Source: CAD feature listing. Evaluate the final solid. Frame: model axes, mm. A direction names the side the tool comes from. Coordinates: 2 decimals unless noted, no trailing zeros. Order: outer loops, then holes, each group sorted by start corner. A loop starts at its lowest first (then second) coordinate and runs counter-clockwise, first axis right, second up.
Item 1: Ray query, line 1 (Z direction, x = -7.75, y = 0); line 2 (Z direction, x = -7, y = -17); line 3 (Y direction, x = -6.5, z = 27). Return the intervals inside material, ascending.
Item 2: Mould query, pull axis Y, two halves, no side actions, for faces 1 (the flat face through (-5, -1, -18)), 2 (the cylindrical face through (-10.07, 36.4, 0.53)), 3 (the cylindrical face through (-11.796, -17.436, -23.172)), 4 (the cylindrical face through (-3.028, -2.05, -15.616)). Classes: released by +Y, released by -Y, zero draft, split by the parting line, or undercut.
Item 3: Section B-B on z = 0. State how many separate pieces and enclosed holes the cut face has, then the cut area to 3 significant figures.
Item 4: Reachability of faces 5 (the cylindrical face through (-10.06, 40.06, -12.62)), 6 (the cylindrical face through (-11.465, -2.05, 15.616)) from +Z, -Z, +X, -X, +Y, -Y: full face, straight path, thin tool, end or side. Return the list, or none.
Item 5: Section A-A on y = 0. Return the cut outline in (x, z), then the cut area to 4 significant figures.
Item 6: Contact query for flat-ended pins moving along their axis: P1, Ø1, axis at y = 25, z = -33, coming from the +X side; P2, Ø3, axis at y = -21, z = -18.5, coming from the -X side; P3, Ø12, axis at y = 15.5, z = -18.5, coming from the -X side; P4, Ø1.5, axis at x = -7.5, z = -22.5, coming from the +Y side. Output: stop coordinate, or through.
Autodesk Inventor part; units mm, degrees
ref_plane "YZ Plane" through (0, 0, 0) normal (1, 0, 0) x (0, 1, 0)
ref_plane "XZ Plane" through (0, 0, 0) normal (0, 1, 0) x (-1, 0, 0)
ref_plane "XY Plane" through (0, 0, 0) normal (0, 0, 1) x (1, 0, 0)
sketch "Sketch1" plane through (0, 0, 0) normal (0, 0, 1) x (1, 0, 0)
  line L0 (-15, 41) -> (-15, 16.75)
  line L1 (-14, 15.75) -> (-9, 15.75)
  line L2 (-9, 15.75) -> (-9, 0)
  line L3 (-9, 0) -> (0, 0)
  line L4 (0, 0) -> (0, 14.75)
  line L5 (-1, 15.75) -> (-5, 15.75)
  line L6 (-5, 15.75) -> (-5, 41)
  line L7 (-6, 42) -> (-14, 42)
  line L8 (-5, 41) -> (-6, 42)
  line L9 (-15, 41) -> (-14, 42)
  line L10 (-14, 15.75) -> (-15, 16.75)
  line L11 (-1, 15.75) -> (0, 14.75)
  point P0 (-15, 42)
  point P1 (-15, 15.75)
  point P2 (0, 15.75)
  point P3 (-5, 42)
  point P4 (0, 7.375)
  point P5 (-4.5, 0)
  point P6 (-10, 42)
  point P7 (-11.5, 15.75)
  dimension "d1" = 6
  dimension "d2" = 15.75
  dimension "d3" = 5
  dimension "d4" = 15
  dimension "d5" = 1
  dimension "d6" = 1
  dimension "d7" = 1
  dimension "d8" = 1
  dimension "d9" = 1
  dimension "d10" = 1
  dimension "d11" = 1
  dimension "d12" = 1
  dimension "d13" = 42
  dimension "d14" = 15.75
revolve "Revolution1" add sketch "Sketch1" angle 360 about axis through (-9, 0, 0) along (1, 0, 0)
sketch "Sketch2" plane through (-5, 0, 0) normal (1, 0, 0) x (0, 0, -1)
  circle A0 centre (0, 0) radius 34
  circle A1 centre (0, 0) radius 30
  circle A2 centre (0, 0) radius 25
  circle A3 centre (0, 34) radius 2.5
  line L0 (0, 0) -> (42, 0)
  circle A4 centre (0, 0) radius 42
  line L1 (27.7164, -11.4805) -> (0, 0)
  point P0 (0, -34)
  point P1 (0, 25)
  point P2 (0, -25)
  point P3 (-25, 0)
  point P4 (25, 0)
  point P5 (-17.6777, 17.6777)
  point P6 (17.6777, -17.6777)
  point P7 (-17.6777, -17.6777)
  point P8 (17.6777, 17.6777)
  dimension "d16" = 68
  dimension "d17" = 60
  dimension "d18" = 50
  dimension "d19" = 5
  dimension "d22" = 360
  dimension "d55" = -22.5
hole "Hole1" at (-5, 34, 0) at (-5, -34, 0) direction (-1, 0, 0) diameter 4.917 depth 10
hole "Hole2" at (-5, 25, 0) at (-5, 0, -25) at (-5, -25, 0) at (-5, 0, 25) direction (-1, 0, 0) diameter 6 end up to surface
hole "Hole3" at (-5, 17.6777, -17.6777) at (-5, -17.6777, -17.6777) at (-5, -17.6777, 17.6777) at (-5, 17.6777, 17.6777) direction (-1, 0, 0) diameter 6.4 end up to surface
hole "Hole5" at (-5, -11.4805, -27.7164) direction (-1, 0, 0) diameter 6 end up to surface
sketch "Sketch4" plane through (-15, 0, 0) normal (-1, 0, 0) x (0, 0, 1)
  circle A0 centre (-17.6777, 17.6777) radius 3.2
  circle A1 centre (-17.6777, 17.6777) radius 5.5
  circle A2 centre (-17.6777, -17.6777) radius 5.5
  circle A3 centre (17.6777, -17.6777) radius 5.5
  circle A4 centre (17.6777, 17.6777) radius 5.5
  point P0 (0, 0)
  dimension "d63" = 11
  dimension "d66" = 360
extrude "Extrusion1" cut sketch "Sketch4" against normal blind 6.5 contours A0 | A1 | A2 | A3 | A4
properties part number "UR5 Gripper Interface plate" material "Aluminum 6061"
Answer list:
1. line 1: z = -42 to -28, -22 to 22, 28 to 42
1. line 2: z = -38.41 to -20.81, -14.55 to 14.55, 20.81 to 38.41
1. line 3: y = -32.17 to -2.24, 2.24 to 32.17
2. face 1: zero draft
2. face 2: undercut
2. face 3: undercut
2. face 4: split by the parting line
3. separate pieces: 5
3. enclosed holes: 0
3. area: 586 mm2
4. face 5: +X, -X
4. face 6: -X
5. outline: (-15, -41) - (-14, -42) - (-6, -42) - (-5, -41) - (-5, -28) - (-15, -28) - close; (-15, -22) - (-5, -22) - (-5, -15.75) - (-1, -15.75) - (0, -14.75) - (0, 14.75) - (-1, 15.75) - (-5, 15.75) - (-5, 22) - (-15, 22) - (-15, 16.75) - (-14, 15.75) - (-9, 15.75) - (-9, -15.75) - (-14, -15.75) - (-15, -16.75) - close; (-15, 28) - (-5, 28) - (-5, 41) - (-6, 42) - (-14, 42) - (-15, 41) - close
5. area: 684.5 mm2
6. P1: stops at x = -5
6. P2: stops at x = -8.5
6. P3: stops at x = -15
6. P4: stops at y = 35.93
